```python
from build123d import *

# Parameters (mm, degrees)
BOSS_EXTRUDE1_DEPTH = 19.05


with BuildPart() as part:
    # Sketch1 → Boss-Extrude1 (new body)
    with BuildSketch(Plane(origin=(0, 0, 0), x_dir=(1, 0, 0), z_dir=(0, 1, 0))):
        Polygon((-55.333344517, 0), (-51.121344464, -21.175154204), (-39.126583134, -39.126583134), (-21.175154204, -51.121344464), (0, -55.333344517), (21.175154204, -51.121344464), (39.126583134, -39.126583134), (51.121344464, -21.175154204), (55.333344517, 0), (51.121344464, 21.175154204), (39.126583134, 39.126583134), (21.175154204, 51.121344464), (0, 55.333344517), (-21.175154204, 51.121344464), (-39.126583134, 39.126583134), (-51.121344464, 21.175154204), align=None)
        Polygon((-35.910132953, 0), (-33.176636845, -13.742212935), (-25.392298524, -25.392298524), (-13.742212935, -33.176636845), (0, -35.910132953), (13.742212935, -33.176636845), (25.392298524, -25.392298524), (33.176636845, -13.742212935), (35.910132953, 0), (33.176636845, 13.742212935), (25.392298524, 25.392298524), (13.742212935, 33.176636845), (0, 35.910132953), (-13.742212935, 33.176636845), (-25.392298524, 25.392298524), (-33.176636845, 13.742212935), align=None, mode=Mode.SUBTRACT)
    extrude(amount=BOSS_EXTRUDE1_DEPTH)

    # Sketch3 → Cut-Revolve1 (revolve, cut)
    with BuildSketch(Plane.XY, mode=Mode.PRIVATE) as cut_revolve1_sk:
        Polygon((-46.636756029, 0), (-44.45, 24.994735789), (-114.963192857, 24.994735789), (-114.963192857, 0), align=None)
    revolve(cut_revolve1_sk.sketch.rotate(Axis((0, 0, 0), (0, 1, 0)), 180), axis=Axis((0, 0, 0), (0, 1, 0)), mode=Mode.SUBTRACT)


solid = part.part
```
Here's how the part is built. I have some questions about the finished solid (model axes, mm). A direction names the side the tool comes from. Give positions to 0.01 mm unless a question says otherwise; leave off trailing zeros. Write each loop counter-clockwise with the first axis right and the second up, starting at its lowest first coordinate (ties: lowest second). Pieces come first, ordered by that corner, then holes. Notation, with made-up numbers: (83, 40) -> (112, 40) arc R30 cw to (112, 73) -> close; hole circle Ø6 at (72, 14). An arc over 180 degrees is marked (long way). Use one line per item in the form item = value.
1) Suppose I cut it at A-A (y = 6.5). Please give me the cut outline in (x, z).
Verdict:
outline = circle Ø92.14 at (0, 0); hole (-35.91, 0) -> (-33.18, -13.74) -> (-25.39, -25.39) -> (-13.74, -33.18) -> (0, -35.91) -> (13.74, -33.18) -> (25.39, -25.39) -> (33.18, -13.74) -> (35.91, 0) -> (33.18, 13.74) -> (25.39, 25.39) -> (13.74, 33.18) -> (0, 35.91) -> (-13.74, 33.18) -> (-25.39, 25.39) -> (-33.18, 13.74) -> close
2) If I drill on L1, parallel to Z at x = -7, y = 15.25; L2, parallel to X at y = 15.75, z = -21.5; L3, parallel to X at y = 17.5, z = 6, over which ranges is the centre line in solid material (lowest first)? Write a range as [from, to].
Verdict:
L1 = [-44.76, -34.52], [34.52, 44.76]
L2 = [-39.83, -27.99], [27.99, 39.83]
L3 = [-44.7, -34.72], [34.72, 44.7]
3) Suppose I cut it at B-B (y = 16.5). Please give me the cut outline in (x, z).
Verdict:
outline = circle Ø90.39 at (0, 0); hole (-35.91, 0) -> (-33.18, -13.74) -> (-25.39, -25.39) -> (-13.74, -33.18) -> (0, -35.91) -> (13.74, -33.18) -> (25.39, -25.39) -> (33.18, -13.74) -> (35.91, 0) -> (33.18, 13.74) -> (25.39, 25.39) -> (13.74, 33.18) -> (0, 35.91) -> (-13.74, 33.18) -> (-25.39, 25.39) -> (-33.18, 13.74) -> close
4) We'd pull the mould along X, two halves only. Please class faces 3 (the face through (-5.913, 13.892, -45.035)), 4 (the face through (6.775, 9.392, 34.563)), 5 (the face through (-7, 0, -35)): +X half, -X half, draft (parallel to the pull), parting line (faces both ways), or undercut.
Verdict:
face_3 = parting line
face_4 = undercut
face_5 = draft
5) On a 3-axis mill with a long thin cutter (end or side, diameter ignored), from which of +Z, -Z, +X, -X, +Y, -Y can I reach the whole of each face in a straight line? I mean faces 1 (the face through (-20, 19.05, 30)), 2 (the face through (-19.65, 9.39, 29.23)). Say none if no direction works.
Verdict:
face_1 = +Z, -Z, +X, -X, +Y
face_2 = +Y, -Y
6) I'm going to push flat-ended pins straight in: pin 1 (4 mm diameter, centred on x = -32.5, y = 4, fed in from +Z); pin 2 (10 mm diameter, centred on y = 4, z = -24.5, fed in from -X); pin 3 (8 mm diameter, centred on y = 16.5, z = 36.5, fed in from +X). Where does each tip first touch, or does it pass through?
Verdict:
pin_1 = 34.83
pin_2 = -42.03
pin_3 = 31.43
